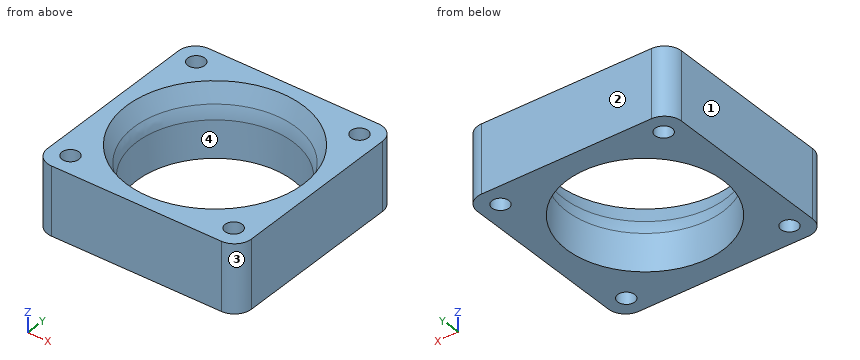
from build123d import *

# Parameters (mm, degrees)
SKETCH1_W           = 30
SKETCH1_H           = 30
BOSS_EXTRUDE1_DEPTH = 10
FILLET1_R           = 2.5
SKETCH2_R           = 1.25
CUT_EXTRUDE1_DEPTH  = 24.452078799
FILLET2_R           = 5


with BuildPart() as part:
    # Sketch1 → Boss-Extrude1 (new body)
    with BuildSketch(Plane.XY):
        Rectangle(SKETCH1_W, SKETCH1_H)
    extrude(amount=BOSS_EXTRUDE1_DEPTH)

    # Fillet1
    fillet1_edges = [part.edges().sort_by_distance(p)[0] for p in [
        (15, -15, 5),
        (-15, -15, 5),
        (-15, 15, 5),
        (15, 15, 5),
    ]]
    fillet(fillet1_edges, radius=FILLET1_R)

    # Sketch2 → Cut-Extrude1 (cut, through all)
    with BuildSketch(Plane.XY.offset(10)):
        with Locations((-12, 12)):
            Circle(SKETCH2_R)
        with Locations((12, 12)):
            Circle(SKETCH2_R)
        with Locations((12, -12)):
            Circle(SKETCH2_R)
        with Locations((-12, -12)):
            Circle(SKETCH2_R)
    extrude(amount=-CUT_EXTRUDE1_DEPTH, mode=Mode.SUBTRACT)

    # Sketch4 → Cut-Revolve1 (revolve, cut)
    with BuildSketch(Plane(origin=(0, 0, 0), x_dir=(0, 0, -1), z_dir=(1, 0, 0)), mode=Mode.PRIVATE) as cut_revolve1_sk:
        Polygon((0, 0), (-10, 0), (-10, 13), (-6.5, 11.5), (0, 11.5), align=None)
    revolve(cut_revolve1_sk.sketch.rotate(Axis((0, 0, 0), (0, 0, 1)), 90), axis=Axis((0, 0, 0), (0, 0, 1)), mode=Mode.SUBTRACT)

    # Fillet2
    fillet2_edges = [part.edges().sort_by_distance(p)[0] for p in [
        (11.5, 0, 6.5),
    ]]
    fillet(fillet2_edges, radius=FILLET2_R)


solid = part.part
Read the model definition and answer for the solid it produces. Units are mm, in the model's axes. Face numbers are marked on the shaded views. Round coordinates to 2 decimals unless told otherwise and drop trailing zeros. Order: outer loops, then holes, each group sorted by start corner. A loop starts at its lowest first (then second) coordinate and runs counter-clockwise, first axis right, second up. Notation, with made-up numbers: (17.25, 73.25) - (74.25, 73.25) arc R24 ccw to (74.25, 111.25) - close; hole circle Ø6 at (48.25, -21.5). An arc over 180 degrees is marked (long way). Use one line per item in the form item = value. Start each with the question number.
(1) The part is cut by section B-B (z = 8.5). Give the vertices of the cut face in (x, y).
(2) Determine the mould class of the marked faces 1, 2, 3 and 4 for opening direction X: +X half, -X half, draft (parallel to the pull), parting line (faces both ways), or undercut.
(3) Find the intervals of material crossed by line 1 along Y through (x, z) = (12, 4); line 2 along Y through (x, z) = (-12.5, 1.75); line 3 along Y through (x, z) = (0, 1.9), in increasing order. Write a range as from..to.
(4) The part is cut by section A-A (z = 1.5). Give the vertices of the cut face in (x, y).
Checked values:
q1.outline = (-15, -12.5) arc R2.5 ccw to (-12.5, -15) - (12.5, -15) arc R2.5 ccw to (15, -12.5) - (15, 12.5) arc R2.5 ccw to (12.5, 15) - (-12.5, 15) arc R2.5 ccw to (-15, 12.5) - close; hole circle Ø2.5 at (-12, -12); hole circle Ø2.5 at (-12, 12); hole circle Ø24.71 at (0, 0); hole circle Ø2.5 at (12, -12); hole circle Ø2.5 at (12, 12)
q2.face_1 = -X half
q2.face_2 = draft
q2.face_3 = +X half
q2.face_4 = undercut
q3.line_1 = -15..-13.25, -10.75..10.75, 13.25..15
q3.line_2 = -15..-13.15, -10.85..10.85, 13.15..15
q3.line_3 = -15..-11.5, 11.5..15
q4.outline = (-15, -12.5) arc R2.5 ccw to (-12.5, -15) - (12.5, -15) arc R2.5 ccw to (15, -12.5) - (15, 12.5) arc R2.5 ccw to (12.5, 15) - (-12.5, 15) arc R2.5 ccw to (-15, 12.5) - close; hole circle Ø2.5 at (-12, -12); hole circle Ø2.5 at (-12, 12); hole circle Ø23 at (0, 0); hole circle Ø2.5 at (12, -12); hole circle Ø2.5 at (12, 12)
